Verification items for the finished model (mm, model axes). A direction names the side the tool comes from. Give positions to 0.01 mm unless a question says otherwise; leave off trailing zeros. Order: outer loops, then holes, each group sorted by start corner. A loop starts at its lowest first (then second) coordinate and runs counter-clockwise, first axis right, second up.
(1) Sectioned sample at B-B on z = 52. Record the cut outline in (x, y).
(2) Sectioned sample at A-A on x = 4. Record the cut outline in (y, z), plus the area to 3 significant figures.
(3) Mould release check, pull along X, two halves, no side actions. Record for faces 3 (the face through (-13.39, 184, 36)), 4 (the face through (-51, 184, 30)), 5 (the face through (-1, 186, 23)): pulls with the +X half, pulls with the -X half, needs draft (parallel to the pull), parting line crosses it, or undercut.
(4) Scan lines: L1, parallel to X at y = 185.15, z = 52; L2, parallel to Z at x = -43, y = 184.5; L3, parallel to X at y = 185.55, z = 41. Record each from-to range of solid material in increasing order.
(5) Access from +Z, -Z, +X, -X, +Y, -Y to the whole of each face (thin tool, end or side, straight path). Record for faces 1 (the face through (-10.679, 184.479, 45.676)), 2 (the face through (-1, 183, 23)).
(6) Sectioned sample at C-C on x = 43. Record the cut outline in (y, z).
(7) Sectioned sample at D-D on y = 184.1. Record the cut outline in (x, z).
```python
from build123d import *

# Parameters (mm, degrees)
SKETCH003_R                = 1.8
EXTRUDE002_DEPTH           = 10
EXTRUDE002_PLACEMENT_ANGLE = 90
CYLINDER002_R              = 1.8
CYLINDER002_DEPTH          = 200
ARRAY_X_COUNT              = 2
ARRAY_X_PITCH              = 86
ARRAY_Z_COUNT              = 2
ARRAY_Z_PITCH              = 44
BOX008_W                   = 102
BOX008_H                   = 3
BOX008_DEPTH               = 60


with BuildPart() as power_input_extrude:
    # Sketch003 → Extrude002 (new body)
    with BuildSketch(Plane.XY):
        with Locations((39.109962, 21.410699)):
            Circle(SKETCH003_R)
        with Locations((79.109962, 21.410699)):
            Circle(SKETCH003_R)
        Polygon((45.609962, 11.910699), (45.609962, 25.910699), (51.109962, 30.910699), (67.109962, 30.910699), (72.609962, 25.910699), (72.609962, 11.910699), align=None)
    extrude(amount=-EXTRUDE002_DEPTH)


with BuildPart() as power_input_extrude_1:
    # Extrude002 placement: moved
    add(power_input_extrude.part.moved(Location((-59, 180, 17.3))).rotate(Axis((-59, 180, 17.3), (1, 0, 0)), EXTRUDE002_PLACEMENT_ANGLE))


with BuildPart() as back_wall_hole_fusion:
    # Cylinder002 → Cylinder002 (new body)
    with BuildSketch(Plane(origin=(-43, 200, 8), x_dir=(1, 0, 0), z_dir=(0, -1, 0))):
        Circle(CYLINDER002_R)
    extrude(amount=CYLINDER002_DEPTH)

    # Array X: back wall hole fusion ×2


with BuildPart() as back_wall_hole_fusion_1:
    add(back_wall_hole_fusion.part)
    with Locations(*[(i * ARRAY_X_PITCH, 0, 0) for i in range(1, ARRAY_X_COUNT)]):
        add(back_wall_hole_fusion.part)

    # Array Z: back wall hole fusion ×2


with BuildPart() as back_wall_hole_fusion_2:
    add(back_wall_hole_fusion_1.part)
    with Locations(*[(0, 0, i * ARRAY_Z_PITCH) for i in range(1, ARRAY_Z_COUNT)]):
        add(back_wall_hole_fusion_1.part)

    # Fusion006: union power input extrude
    add(power_input_extrude_1.part)


with BuildPart() as back_wall_cut:
    # Box008 → Box008 (new body)
    with BuildSketch(Plane(origin=(-51, 183, 0), x_dir=(1, 0, 0), z_dir=(0, 0, 1))):
        with Locations((51, 1.5)):
            Rectangle(BOX008_W, BOX008_H)
    extrude(amount=BOX008_DEPTH)

    # Cut009: cut back wall hole fusion
    add(back_wall_hole_fusion_2.part, mode=Mode.SUBTRACT)


solid = back_wall_cut.part
```
Ans:
1. outline: (-51, 183) - (-44.8, 183) - (-44.8, 186) - (-51, 186) - close; (-41.2, 183) - (41.2, 183) - (41.2, 186) - (-41.2, 186) - close; (44.8, 183) - (51, 183) - (51, 186) - (44.8, 186) - close
2. outline: (183, 0) - (186, 0) - (186, 29.21) - (183, 29.21) - close; (183, 48.21) - (186, 48.21) - (186, 60) - (183, 60) - close
2. area: 123 mm2
3. face 3: undercut
3. face 4: pulls with the -X half
3. face 5: needs draft
4. L1: x = -51 to -44.8, -41.2 to 41.2, 44.8 to 51
4. L2: z = 0 to 6.2, 9.8 to 50.2, 53.8 to 60
4. L3: x = -51 to -13.39, 13.61 to 51
5. face 1: +Y, -Y
5. face 2: +Z, -Z, +X, -X, -Y
6. outline: (183, 0) - (186, 0) - (186, 6.2) - (183, 6.2) - close; (183, 9.8) - (186, 9.8) - (186, 50.2) - (183, 50.2) - close; (183, 53.8) - (186, 53.8) - (186, 60) - (183, 60) - close
7. outline: (-51, 0) - (51, 0) - (51, 60) - (-51, 60) - close; hole circle Ø3.6 at (-43, 8); hole circle Ø3.6 at (-43, 52); hole circle Ø3.6 at (-19.89, 38.71); hole (-13.39, 29.21) - (13.61, 29.21) - (13.61, 43.21) - (8.11, 48.21) - (-7.89, 48.21) - (-13.39, 43.21) - close; hole circle Ø3.6 at (20.11, 38.71); hole circle Ø3.6 at (43, 8); hole circle Ø3.6 at (43, 52)
